```python
from build123d import *

# Parameters (mm, degrees)
F0_W      = 24
F0_H      = 56
F0_W_2    = 17
F0_H_2    = 38
F1_DEPTH  = 35
F2_R      = 1.5
F3_DEPTH  = 15
F4_R      = 3
F6_DEPTH  = 5
F7_R      = 5
F8_DEPTH  = 25
F9_R      = 2
F10_DEPTH = 25
F11_R     = 6
F12_DEPTH = 2
F13_R     = 7
F14_DEPTH = 4


with BuildPart() as f1:
    # F0 (on Top) → F1 (new body)
    with BuildSketch(Plane.XY):
        with Locations((12, 28)):
            Rectangle(F0_W, F0_H)
        with Locations((12, 28)):
            Rectangle(F0_W_2, F0_H_2, mode=Mode.SUBTRACT)
    extrude(amount=F1_DEPTH)

    # F2 (on face) → F3 (cut)
    with BuildSketch(Plane.XY.offset(35)):
        with Locations((12, 49.5)):
            Circle(F2_R)
        with Locations((12, 6.5)):
            Circle(F2_R)
    extrude(amount=-F3_DEPTH, mode=Mode.SUBTRACT)

    # F4
    f4_edges = [f1.edges().sort_by_distance(p)[0] for p in [
        (24, 0, 17.5),
        (24, 56, 17.5),
    ]]
    fillet(f4_edges, radius=F4_R)

    # F5 (on face) → F6 (join)
    with BuildSketch(Plane(origin=(0, 0, 0), x_dir=(1, 0, 0), z_dir=(0, 0, -1))):
        with BuildLine():
            Line((21, 0), (0, 0))
            Line((0, 0), (0, -56))
            Line((0, -56), (21, -56))
            ThreePointArc((21, -56), (23.12132, -55.12132), (24, -53))
            Line((24, -53), (24, -3))
            ThreePointArc((24, -3), (23.12132, -0.87868), (21, 0))
        make_face()
    extrude(amount=F6_DEPTH)

    # F7 (on face) → F8 (cut)
    with BuildSketch(Plane.XY):
        with Locations((12, 37)):
            Circle(F7_R)
    extrude(amount=-F8_DEPTH, mode=Mode.SUBTRACT)

    # F9 (on face) → F10 (cut)
    with BuildSketch(Plane(origin=(0, 0, 0), x_dir=(0, -1, 0), z_dir=(-1, 0, 0))):
        with Locations((-51, 13)):
            Circle(F9_R)
        with Locations((-5, 13)):
            Circle(F9_R)
    extrude(amount=-F10_DEPTH, mode=Mode.SUBTRACT)

    # F11 (on face) → F12 (cut)
    with BuildSketch(Plane.YZ.offset(24)):
        with Locations((5, 13)):
            Circle(F11_R)
        with Locations((51, 13)):
            Circle(F11_R)
    extrude(amount=-F12_DEPTH, mode=Mode.SUBTRACT)

    # F13 (on face) → F14 (cut)
    with BuildSketch(Plane(origin=(0, 0, 0), x_dir=(0, -1, 0), z_dir=(-1, 0, 0))):
        with Locations((-28.088422, 11)):
            Circle(F13_R)
    extrude(amount=-F14_DEPTH, mode=Mode.SUBTRACT)


solid = f1.part
```
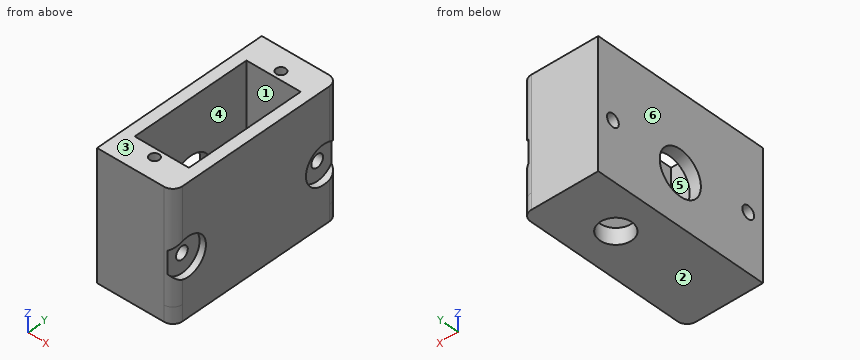
Geometry: final body of the model. Coordinates: model frame, mm. Face numbers are marked on the shaded views. A direction names the side the tool comes from. Coordinates: 2 decimals unless noted, no trailing zeros. Order: outer loops, then holes, each group sorted by start corner. A loop starts at its lowest first (then second) coordinate and runs counter-clockwise, first axis right, second up. Notation, with made-up numbers: (26.25, 63) -> (38.25, 63) arc R29 cw to (38.25, 94) -> close; hole circle Ø9 at (-14.75, -28). An arc over 180 degrees is marked (long way). Answer in a Markdown table with one row per item.
Item 1: Contact query for flat-ended pins moving along their axis: P1, Ø0.9, axis at x = 11.5, y = 6, coming from the +Z side; P2, Ø11.5, axis at x = 12, y = 37, coming from the +Z side. Output: stop coordinate, or through.
Return value:
| item | result |
|---|---|
| P1 | stops at z = 20 |
| P2 | stops at z = 0 |
Item 2: Ray query, L1, parallel to X at y = 20, z = 33.5; L2, parallel to Y at x = 12.5, z = 9.5; L3, parallel to Y at x = 4.5, z = 12. Return the intervals inside material, ascending.
Return value:
| item | result |
|---|---|
| L1 | x = 0 to 3.5, 20.5 to 24 |
| L2 | y = 0 to 9, 47 to 56 |
| L3 | y = 0 to 3.27, 6.73 to 9, 47 to 49.27, 52.73 to 56 |
Item 3: Section C-C on x = 15.5. Output: boundary loops of the cut face in (y, z).
Return value:
| item | result |
|---|---|
| outline | (0, -5) -> (33.43, -5) -> (33.43, 0) -> (9, 0) -> (9, 35) -> (0, 35) -> close; (40.57, -5) -> (56, -5) -> (56, 35) -> (47, 35) -> (47, 0) -> (40.57, 0) -> close; hole circle Ø4 at (5, 13); hole circle Ø4 at (51, 13) |
Item 4: Access query for the marked faces 1 and 2. Directions: +Z, -Z, +X, -X, +Y, -Y. A direction counts if a zero-diameter tool reaches every point of the face in a straight line with its end or side. Return the directions, or none.
Return value:
| item | result |
|---|---|
| face 1 | +Z |
| face 2 | -Z, +X, -X, +Y, -Y |
Item 5: Section A-A on y = 37. Output: boundary loops of the cut face in (x, z), plus the area to 3 significant figures.
Return value:
| item | result |
|---|---|
| outline | (0, -5) -> (7, -5) -> (7, 0) -> (3.5, 0) -> (3.5, 35) -> (0, 35) -> close; (17, -5) -> (24, -5) -> (24, 35) -> (20.5, 35) -> (20.5, 0) -> (17, 0) -> close |
| area | 315 mm² |
Item 6: Draft query along X for the marked faces 3, 4, 5 and 6. Return one class per face: released by +X, released by -X, zero draft, split by the parting line, or undercut.
Return value:
| item | result |
|---|---|
| face 3 | zero draft |
| face 4 | undercut |
| face 5 | undercut |
| face 6 | released by -X |
Item 7: Section D-D on x = 18.75. Output: boundary loops of the cut face in (y, z), plus the area to 3 significant figures.
Return value:
| item | result |
|---|---|
| outline | (0, -5) -> (56, -5) -> (56, 35) -> (47, 35) -> (47, 0) -> (9, 0) -> (9, 35) -> (0, 35) -> close; hole circle Ø4 at (5, 13); hole circle Ø4 at (51, 13) |
| area | 885 mm² |
Item 8: Section B-B on x = 2. Output: boundary loops of the cut face in (y, z).
Return value:
| item | result |
|---|---|
| outline | (0, -5) -> (56, -5) -> (56, 35) -> (0, 35) -> close; hole circle Ø4 at (5, 13); hole circle Ø14 at (28.09, 11); hole circle Ø4 at (51, 13) |
